Geometry check sheet. Reference: the model listing, model coordinates, mm. A direction names the side the tool comes from. Coordinates: 2 decimals unless noted, no trailing zeros. Write each loop counter-clockwise with the first axis right and the second up, starting at its lowest first coordinate (ties: lowest second). Pieces come first, ordered by that corner, then holes. Notation, with made-up numbers: (4.5, 5) -> (11.5, 5) arc R21 ccw to (11.5, 36) -> close; hole circle Ø9 at (30.25, 51). An arc over 180 degrees is marked (long way). Use a Markdown table: item, result.
```python
from build123d import *

# Parameters (mm, degrees)
BOSS_EXTRUDE1_DEPTH = 5
FILLET1_R           = 1
SKETCH3_R           = 1.6
SKETCH3_R_2         = 2
CUT_EXTRUDE1_DEPTH  = 26.465387384


with BuildPart() as part:
    # Sketch1 → Boss-Extrude1 (new, symmetric)
    with BuildSketch(Plane(origin=(0, 0, 0), x_dir=(0, 0, -1), z_dir=(1, 0, 0))):
        with BuildLine():
            Line((-3, -7.416198487), (-3, -22.416198487))
            Line((-3, -22.416198487), (-1, -22.416198487))
            Line((-1, -22.416198487), (-1, -6.017474553))
            ThreePointArc((-1, -6.017474553), (0, 6.1), (1, -6.017474553))
            Line((1, -6.017474553), (1, -22.416198487))
            Line((1, -22.416198487), (3, -22.416198487))
            Line((3, -22.416198487), (3, -7.416198487))
            ThreePointArc((3, -7.416198487), (0, 8), (-3, -7.416198487))
        make_face()
    extrude(amount=BOSS_EXTRUDE1_DEPTH, both=True)

    # Fillet1
    fillet1_edges = [part.edges().sort_by_distance(p)[0] for p in [
        (0, -6.017474553, 1),
        (0, -7.416198487, 3),
        (0, -7.416198487, -3),
        (0, -6.017474553, -1),
    ]]
    fillet(fillet1_edges, radius=FILLET1_R)

    # Sketch3 → Cut-Extrude1 (cut, through all)
    with BuildSketch(Plane.XY.offset(3)):
        with Locations((0, -19.666198487)):
            Circle(SKETCH3_R)
        with Locations((0, -11.062257748)):
            Circle(SKETCH3_R_2)
    extrude(amount=-CUT_EXTRUDE1_DEPTH, mode=Mode.SUBTRACT)


solid = part.part
```
Item 1: Section check D-D on y = -10.5. Record the boundary of the cut face in (x, z), then the cut area to 3 significant figures.
Answer block:
| item | result |
|---|---|
| outline | (-5, -3) -> (-1.92, -3) -> (-1.92, -1) -> (-5, -1) -> close; (-5, 1) -> (-1.92, 1) -> (-1.92, 3) -> (-5, 3) -> close; (1.92, -3) -> (5, -3) -> (5, -1) -> (1.92, -1) -> close; (1.92, 1) -> (5, 1) -> (5, 3) -> (1.92, 3) -> close |
| area | 24.6 mm^2 |
Item 2: Mould release check, pull along Y, two halves, no side actions. Record for faces 4 (the cylindrical face through (0, 8, 0)), 5 (the flat face through (5, -7.1, 1.2)), 6 (the cylindrical face through (-0.26, -9.08, -1.99)), 7 (the flat face through (0, -22.416, -2)): +Y half, -Y half, draft (parallel to the pull), parting line (faces both ways), or undercut.
Answer block:
| item | result |
|---|---|
| face 4 | parting line |
| face 5 | draft |
| face 6 | undercut |
| face 7 | -Y half |
Item 3: Thickness scan on L1, parallel to Y at x = 0, z = -2.55; L2, parallel to Z at x = 2.5, y = 0; L3, parallel to Z at x = 2, y = -17. Record the ranges inside material, lowest first. Write a range as [from, to].
Answer block:
| item | result |
|---|---|
| L1 | y = [-22.42, -21.27], [-18.07, -13.06], [-9.06, -5.54], [5.54, 7.58] |
| L2 | z = [-8, -6.1], [6.1, 8] |
| L3 | z = [-3, -1], [1, 3] |
Item 4: Depth check by flat-ended pin: P1, Ø5, axis at x = -2, y = -14, coming from the -Z side; P2, Ø3, axis at x = -1.5, y = -12, coming from the +Z side; P3, Ø3, axis at x = 0.5, z = -0.5, coming from the +Y side; P4, Ø1, axis at x = -2, z = 1.5, coming from the +Y side. Enter the tip coordinate at first touch or a pass-through.
Answer block:
| item | result |
|---|---|
| P1 | stops at z = -3 |
| P2 | stops at z = 3 |
| P3 | stops at y = 8 |
| P4 | stops at y = 7.94 |
Item 5: Section check C-C on z = 5.5. Record the boundary of the cut face in (x, y), then the cut area to 3 significant figures.
Answer block:
| item | result |
|---|---|
| outline | (-5, -5.81) -> (5, -5.81) -> (5, -2.64) -> (-5, -2.64) -> close; (-5, 2.64) -> (5, 2.64) -> (5, 5.81) -> (-5, 5.81) -> close |
| area | 63.4 mm^2 |
Item 6: Section check B-B on y = 0. Record the boundary of the cut face in (x, z).
Answer block:
| item | result |
|---|---|
| outline | (-5, -8) -> (5, -8) -> (5, -6.1) -> (-5, -6.1) -> close; (-5, 6.1) -> (5, 6.1) -> (5, 8) -> (-5, 8) -> close |
Item 7: Tool access check on faces 1 (the flat face through (0, -15, 3)), 2 (the flat face through (0, -15, -1)), 3 (the cylindrical face through (0.07, -6.21, 1.2)). Record the directions out of +Z, -Z, +X, -X, +Y, -Y that give a thin tool (end or side, any length) a straight path to the whole face; none if there is none.
Answer block:
| item | result |
|---|---|
| face 1 | +Z, +X, -X, -Y |
| face 2 | +X, -X, -Y |
| face 3 | +X, -X |
Item 8: Section check A-A on x = 0. Record the boundary of the cut face in (y, z), then the cut area to 3 significant figures.
Answer block:
| item | result |
|---|---|
| outline | (-22.42, -3) -> (-21.27, -3) -> (-21.27, -1) -> (-22.42, -1) -> close; (-22.42, 1) -> (-21.27, 1) -> (-21.27, 3) -> (-22.42, 3) -> close; (-18.07, -3) -> (-13.06, -3) -> (-13.06, -1) -> (-18.07, -1) -> close; (-18.07, 1) -> (-13.06, 1) -> (-13.06, 3) -> (-18.07, 3) -> close; (-9.06, -3) -> (-8.06, -3) arc R1 cw to (-7.17, -3.56) arc R8 ccw (long way) to (-7.17, 3.56) arc R1 cw to (-8.06, 3) -> (-9.06, 3) -> (-9.06, 1) -> (-6.81, 1) arc R1 ccw to (-5.85, 1.72) arc R6.1 cw (long way) to (-5.85, -1.72) arc R1 ccw to (-6.81, -1) -> (-9.06, -1) -> close |
| area | 110 mm^2 |
